```python
from build123d import *

# Parameters (mm, degrees)
F0_R     = 63.5
F1_DEPTH = 127
F1_TAPER = -20
F2_SIZE  = 63.5
F3_R     = 25.4


with BuildPart() as f1:
    # F0 (on Front) → F1 (new body, symmetric)
    with BuildSketch(Plane.XZ):
        Circle(F0_R)
    extrude(amount=F1_DEPTH, both=True, taper=F1_TAPER)

    # F2
    f2_edges = [f1.edges().sort_by_distance(p)[0] for p in [
        (-109.72422, 127, 0),
    ]]
    chamfer(f2_edges, length=F2_SIZE)

    # F3
    f3_edges = [f1.edges().sort_by_distance(p)[0] for p in [
        (-109.72422, -127, 0),
    ]]
    fillet(f3_edges, radius=F3_R)


solid = f1.part
```
For this review, take the finished solid that the model builds, in its own axes (mm). A direction names the side the tool comes from. Coordinates: 2 decimals unless noted, no trailing zeros. Write each loop counter-clockwise with the first axis right and the second up, starting at its lowest first coordinate (ties: lowest second). Pieces come first, ordered by that corner, then holes. Notation, with made-up numbers: (78, 0.5) - (130, 0.5) arc R25 cw to (130, 30.5) - close; hole circle Ø9 at (61, 68.25). An arc over 180 degrees is marked (long way). Put each result on its own line as item: value.
1. Add section C-C, the plane y = 15. Give the boundary of the cut face in (x, z).
Values found:
outline: circle Ø137.92 at (0, 0)
2. Add section A-A, the plane x = 0. Give the boundary of the cut face in (y, z).
Values found:
outline: (-127, -73.45) arc R25.4 ccw to (-92.91, -97.32) - (0, -63.5) - (67.33, -88.01) - (127, -46.22) - (127, 46.22) - (67.33, 88.01) - (0, 63.5) - (-92.91, 97.32) arc R25.4 ccw to (-127, 73.45) - close
3. Add section B-B, the plane y = 102. Give the boundary of the cut face in (x, z), then the cut area to 3 significant figures.
Values found:
outline: circle Ø127.46 at (0, 0)
area: 12,800 mm²
4. Machinability: for faces 4 (the conical face through (-14.688, 11.693, -66.145)), 5 (the conical face through (46.025, 124.103, 14.494)), which of the approach directions +Z, -Z, +X, -X, +Y, -Y give a long, thin tool a straight path to every point of the face, cutting with its end or side? Answer none if there is none.
Values found:
face 4: none
face 5: +Y
5. For pin 1 (10 mm diameter, centred on x = -56.5, y = -85.5, fed in from -Z); pin 2 (4 mm diameter, centred on x = 23, y = 65.5, fed in from +Z); pin 3 (10 mm diameter, centred on x = 67, z = -52.5, fed in from -Y), all flat-tipped, find the tip position at first contact; note any pin that passes through.
Values found:
pin 1: z = -80.03
pin 2: z = 85.18
pin 3: y = -126.11
6. Mouldability with a two-part tool opening along Y and no side actions: class faces 1 (the conical face through (66.17, -16.14, 20.84)), 2 (the flat face through (-1, -127, 1)), 3 (the flat face through (-1, 127, 1)) as released by +Y, released by -Y, zero draft, split by the parting line, or undercut.
Values found:
face 1: undercut
face 2: released by -Y
face 3: released by +Y
7. Wall thickness on probe 1 along Y at (x, z) = (35, 75); probe 2 along X at (y, z) = (-102.5, -3); probe 3 along Y at (x, z) = (-72.5, -35): over which ranges is each line inside the solid? List them lowest first.
Values found:
probe 1: -125.23 to -52.93, 52.93 to 74.81
probe 2: -98.79 to 98.79
probe 3: -126 to -46.72, 46.72 to 78.04
